Part model, mm, in its own coordinate system. Face numbers are marked on the shaded views. A direction names the side the tool comes from. Coordinates: 2 decimals unless noted, no trailing zeros. Order: outer loops, then holes, each group sorted by start corner. A loop starts at its lowest first (then second) coordinate and runs counter-clockwise, first axis right, second up.
1) Cut at B-B (y = -24). Give the number of separate pieces and of enclosed holes in the cut face, and give its area (3 significant figures).
2) Mould opens along Y. For the marked faces 5, 6 and 7 say: +Y half, -Y half, draft (parallel to the pull), parting line (faces both ways), or undercut.
3) Wall check: L1, parallel to X at y = 30.3, z = 12; L2, parallel to X at y = 16.5, z = 2.5; L3, parallel to Y at x = -15.5, z = 10. Give the ranges that are in metal, low to high.
4) Cut at A-A (x = -15). List the corners of the cut face in (y, z).
5) Tool access for the marked faces 1, 2, 3 and 4: list every direction of +Z, -Z, +X, -X, +Y, -Y with a clear straight run to the whole face (end or side of a thin tool).
6) Cut at D-D (y = -15). List the corners of the cut face in (x, z).
7) Pin check, flat tips, straight feed: pin 1 Ø6.5 at (x, y) = (35, -24) entering from -Z; pin 2 Ø6.5 at (x, y) = (45, -24) entering from +Z; pin 3 Ø3 at (y, z) = (23.5, 16) entering from -X; pin 4 Ø3.5 at (x, y) = (-35, 24) entering from -Z. Stop position of each tip, or through.
8) Cut at C-C (x = 40). List the corners of the cut face in (y, z).
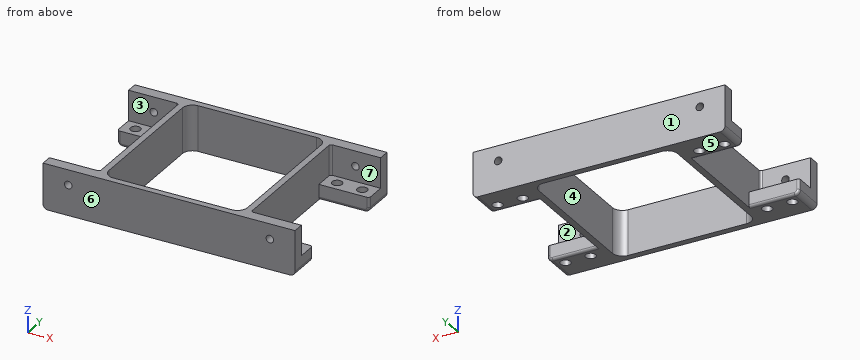
```python
from build123d import *

# Parameters (mm, degrees)
SKETCH_1_W          = 100
SKETCH_1_H          = 65
EXTRUDE_1_DEPTH     = 18
SKETCH_2_W          = 55
SKETCH_2_H          = 60
CUT_EXTRUDE_1_DEPTH = 63.291652731
SKETCH_3_W          = 20
SKETCH_3_H          = 56
CUT_EXTRUDE_2_DEPTH = 12
SKETCH_4_W          = 20
SKETCH_4_H          = 40
CUT_EXTRUDE_3_DEPTH = 61.829680256
SKETCH_5_R          = 2
CUT_EXTRUDE_4_DEPTH = 61.829680256
SKETCH_6_R          = 1.5
CUT_EXTRUDE_5_DEPTH = 84.958322994
FILLET_1_R          = 4
FILLET_2_R          = 2
FILLET_3_R          = 1


with BuildPart() as part:
    # 草图1 → 凸台-拉伸1 (new body)
    with BuildSketch(Plane.XY):
        Rectangle(SKETCH_1_W, SKETCH_1_H)
    extrude(amount=EXTRUDE_1_DEPTH)

    # 草图2 → 切除-拉伸1 (cut, through all)
    with BuildSketch(Plane.XY.offset(18)):
        Rectangle(SKETCH_2_W, SKETCH_2_H)
    extrude(amount=-CUT_EXTRUDE_1_DEPTH, mode=Mode.SUBTRACT)

    # 草图3 → 切除-拉伸2 (cut)
    with BuildSketch(Plane.XY.offset(18)):
        with Locations((40, 0)):
            Rectangle(SKETCH_3_W, SKETCH_3_H)
    cut_extrude_2 = extrude(amount=-CUT_EXTRUDE_2_DEPTH, mode=Mode.SUBTRACT)

    # 草图4 → 切除-拉伸3 (cut, through all)
    with BuildSketch(Plane.XY.offset(6)):
        with Locations((40, 0)):
            Rectangle(SKETCH_4_W, SKETCH_4_H)
    cut_extrude_3 = extrude(amount=-CUT_EXTRUDE_3_DEPTH, mode=Mode.SUBTRACT)

    # 草图5 → 切除-拉伸4 (cut, through all)
    with BuildSketch(Plane.XY.offset(6)):
        with Locations((45, 24)):
            Circle(SKETCH_5_R)
        with Locations((35, 24)):
            Circle(SKETCH_5_R)
        with Locations(Location((35, -24, 0), (0, 0, 180))):
            Circle(SKETCH_5_R)
        with Locations(Location((45, -24, 0), (0, 0, 180))):
            Circle(SKETCH_5_R)
    cut_extrude_4 = extrude(amount=-CUT_EXTRUDE_4_DEPTH, mode=Mode.SUBTRACT)

    # 草图6 → 切除-拉伸5 (cut, through all)
    with BuildSketch(Plane(origin=(0, 32.5, 0), x_dir=(1, 0, 0), z_dir=(0, 1, 0))):
        with Locations(Location((40, -12, 0), (0, 0, 270))):
            Circle(SKETCH_6_R)
    cut_extrude_5 = extrude(amount=-CUT_EXTRUDE_5_DEPTH, mode=Mode.SUBTRACT)

    # 镜向1: 切除-拉伸2, 切除-拉伸3, 切除-拉伸4, 切除-拉伸5 across plane
    add(cut_extrude_2.mirror(Plane(origin=(0, 0, 0), x_dir=(0, 0, 1), z_dir=(1, 0, 0))), mode=Mode.SUBTRACT)
    add(cut_extrude_3.mirror(Plane(origin=(0, 0, 0), x_dir=(0, 0, 1), z_dir=(1, 0, 0))), mode=Mode.SUBTRACT)
    add(cut_extrude_4.mirror(Plane(origin=(0, 0, 0), x_dir=(0, 0, 1), z_dir=(1, 0, 0))), mode=Mode.SUBTRACT)
    add(cut_extrude_5.mirror(Plane(origin=(0, 0, 0), x_dir=(0, 0, 1), z_dir=(1, 0, 0))), mode=Mode.SUBTRACT)

    # 圆角1
    fillet_1_edges = [part.edges().sort_by_distance(p)[0] for p in [
        (27.5, 30, 9),
        (27.5, -30, 9),
        (-27.5, -30, 9),
        (-27.5, 30, 9),
    ]]
    fillet(fillet_1_edges, radius=FILLET_1_R)

    # 圆角2
    fillet_2_edges = [part.edges().sort_by_distance(p)[0] for p in [
        (50, 26.25, 0),
        (-50, 26.25, 0),
        (50, -26.25, 0),
        (-50, -26.25, 0),
    ]]
    fillet(fillet_2_edges, radius=FILLET_2_R)

    # 圆角3
    fillet_3_edges = [part.edges().sort_by_distance(p)[0] for p in [
        (-39, -20, 0),
        (-50, -20, 4),
        (-39, 20, 0),
        (39, 20, 0),
        (-49.414213562, -20, 0.585786438),
        (-50, 20, 4),
        (-49.414213562, 20, 0.585786438),
        (50, -20, 4),
        (49.414213562, -20, 0.585786438),
        (50, 20, 4),
        (49.414213562, 20, 0.585786438),
        (30, 28, 12),
        (30, -28, 12),
        (39, -20, 0),
        (-30, 28, 12),
        (-30, -28, 12),
    ]]
    fillet(fillet_3_edges, radius=FILLET_3_R)


solid = part.part
```
Geometry check:
1. separate pieces: 6
1. enclosed holes: 0
1. area: 232 mm2
2. face 5: draft
2. face 6: -Y half
2. face 7: undercut
3. L1: x = -50 to -41.5, -38.5 to 38.5, 41.5 to 50
3. L2: x = -30 to -27.5, 27.5 to 30
3. L3: y = -32.5 to -30, 30 to 32.5
4. outline: (-32.5, 0) - (-30, 0) - (-30, 18) - (-32.5, 18) - close; (30, 0) - (32.5, 0) - (32.5, 18) - (30, 18) - close
5. face 1: +Z, -Z, +X, -X, +Y
5. face 2: +Z, +X
5. face 3: +Z, -X
5. face 4: +Z, -Z
6. outline: (-30, 0) - (-27.5, 0) - (-27.5, 18) - (-30, 18) - close; (27.5, 0) - (30, 0) - (30, 18) - (27.5, 18) - close
7. pin 1: stops at z = 0
7. pin 2: stops at z = 6
7. pin 3: stops at x = -30
7. pin 4: passes through
8. outline: (-32.5, 0) - (-21, 0) arc R1 ccw to (-20, 1) - (-20, 6) - (-28, 6) - (-28, 10.5) - (-32.5, 10.5) - close; (-32.5, 13.5) - (-28, 13.5) - (-28, 18) - (-32.5, 18) - close; (20, 1) arc R1 ccw to (21, 0) - (32.5, 0) - (32.5, 10.5) - (28, 10.5) - (28, 6) - (20, 6) - close; (28, 13.5) - (32.5, 13.5) - (32.5, 18) - (28, 18) - close
